```python
from build123d import *

# Parameters (mm, degrees)
CUT_EXTRUDE1_REACH = 8
SKETCH2_R          = 2.05


with BuildPart() as part:
    # Sketch1 → Revolve1 (revolve)
    with BuildSketch(Plane.XY):
        Polygon((0, 6), (6.5, 6), (6.5, 5.4), (4.75, 3), (6.5, 0.6), (6.5, 0), (0, 0), align=None)
    revolve(axis=Axis((0, 0, 0), (0, 1, 0)))

    # Sketch2 → Cut-Extrude1 (cut, up to next)
    with BuildSketch(Plane(origin=(0, 6, 0), x_dir=(1, 0, 0), z_dir=(0, 1, 0)), mode=Mode.PRIVATE) as cut_extrude1_sk1:
        Circle(SKETCH2_R)
    cut_extrude1_tool1 = extrude(cut_extrude1_sk1.sketch, amount=-CUT_EXTRUDE1_REACH, mode=Mode.PRIVATE) & part.part
    add(cut_extrude1_tool1.solids().sort_by_distance((0, 6, 0))[0], mode=Mode.SUBTRACT)


solid = part.part
```
Could you check a few things on this model? Use its own coordinates, in mm. A direction names the side the tool comes from. Coordinates: 2 decimals unless noted, no trailing zeros. Write each loop counter-clockwise with the first axis right and the second up, starting at its lowest first coordinate (ties: lowest second). Pieces come first, ordered by that corner, then holes. Notation, with made-up numbers: M -22.75,23.5 L 23.25,23.5 A26 cw 23.25,39.5 Z; hole C 78,78.5 d1. An arc over 180 degrees is marked long. Answer as CSV lines item,"result". Start each with the question number.
1) I want a section at D-D, the plane y = 4.55. Please give me the cut outline in (x, z).
2) I want a section at A-A, the plane z = 0. Please give me the cut outline in (x, y), and give its area (3 significant figures).
3) We'd pull the mould along Z, two halves only. Please class faces 1 (the cylindrical face through (-0.267, 3.042, -2.033)), 2 (the cylindrical face through (-5.158, 5.696, 3.955)), 3 (the flat face through (-2, 0, -2)): +Z half, -Z half, draft (parallel to the pull), parting line (faces both ways), or undercut.
4) I want a section at C-C, the plane y = 1.25. Please give me the cut outline in (x, z), and give its area (3 significant figures).
5) I want a section at B-B, the plane x = 0. Please give me the cut outline in (y, z), and give its area (3 significant figures).
6) For P1, Ø1.5, axis at y = 3.5, z = 0, coming from the -X side; P2, Ø1, axis at x = 2.5, y = 0.5, coming from the -Z side, each with a flat end and sliding along its axis, tell me the tip position at first contact or that it passes through.
7) For faces 4 (the conical face through (-1.053, 2.85, 4.744)), 5 (the cylindrical face through (-5.158, 0.296, 3.955)), which set-ups out of +Z, -Z, +X, -X, +Y, -Y let a thin tool reach every point of the face, with its end or its side?
8) Please list where these lines run through material, in increasing order: line 1 (Y direction, x = -3.75, z = 4.25); line 2 (Z direction, x = 0, y = 2); line 3 (Z direction, x = 1.25, y = 5.8). Write a range as from..to.
Data:
1,outline,"C 0,0 d11.76; hole C 0,0 d4.1"
2,outline,"M -6.5,0 L -2.05,0 L -2.05,6 L -6.5,6 L -6.5,5.4 L -4.75,3 L -6.5,0.6 Z; M 2.05,0 L 6.5,0 L 6.5,0.6 L 4.75,3 L 6.5,5.4 L 6.5,6 L 2.05,6 Z"
2,area,"45.0 mm^2"
3,face 1,"undercut"
3,face 2,"parting line"
3,face 3,"draft"
4,outline,"C 0,0 d12.05; hole C 0,0 d4.1"
4,area,"101 mm^2"
5,outline,"M 0,-6.5 L 0.6,-6.5 L 3,-4.75 L 5.4,-6.5 L 6,-6.5 L 6,-2.05 L 0,-2.05 Z; M 0,2.05 L 6,2.05 L 6,6.5 L 5.4,6.5 L 3,4.75 L 0.6,6.5 L 0,6.5 Z"
5,area,"45.0 mm^2"
6,P1,"stops at x = -5.66"
6,P2,"stops at z = -6.18"
7,face 4,"none"
7,face 5,"+Y, -Y"
8,line 1,"y = 0..1.74, 4.26..6"
8,line 2,"z = -5.48..-2.05, 2.05..5.48"
8,line 3,"z = -6.38..-1.62, 1.62..6.38"
